The figure shows three views and two pictorial views of one solid part (mm, origin at its lowest corner). Answer the questions. A direction names the side the tool comes from. Round coordinates to 2 decimals unless told otherwise and drop trailing zeros. Order: outer loops, then holes, each group sorted by start corner. A loop starts at its lowest first (then second) coordinate and runs counter-clockwise, first axis right, second up. Notation, with made-up numbers: (60.25, 1) -> (97.25, 1) arc R14 cw to (97.25, 17) -> close; hole circle Ø9 at (9.5, 12.5). An arc over 180 degrees is marked (long way). Return JSON: item names as keys, results as strings. Group by question number.
(1) The part is cut by section B-B (z = 17.75). Determine the outline of the cut face in (x, y).
(2) The part is cut by section A-A (y = 67.5). Count the separate pieces of the cut face and the enclosed holes in it, plus the area to 3 significant figures.
(3) Consider line 1 (X direction, y = 57.15, z = 13.5); line 2 (Y direction, x = 19.05, z = 12.25); line 3 (Y direction, x = 37.5, z = 1.5). Determine where each line is inside the solid, lowest interval first. Write a range as [from, to].
(4) Each of these flat-tipped pins is pushed along its axis until it touches: pin 1 (10 mm diameter, centred on y = 40.5, z = 6, fed in from -X); pin 2 (15 mm diameter, centred on x = 19.05, y = 57.15, fed in from +Z); pin 3 (1.6 mm diameter, centred on y = 31.5, z = 1.5, fed in from +X); pin 4 (17 mm diameter, centred on x = 57, y = 32.5, fed in from -Z) (3 decimals). Where does it stop, or does it pass through?
(5) Which of the six approach directions +Z, -Z, +X, -X, +Y, -Y give full straight-line access (tool end or side, diameter ignored) to the marked faces 1 and 2?
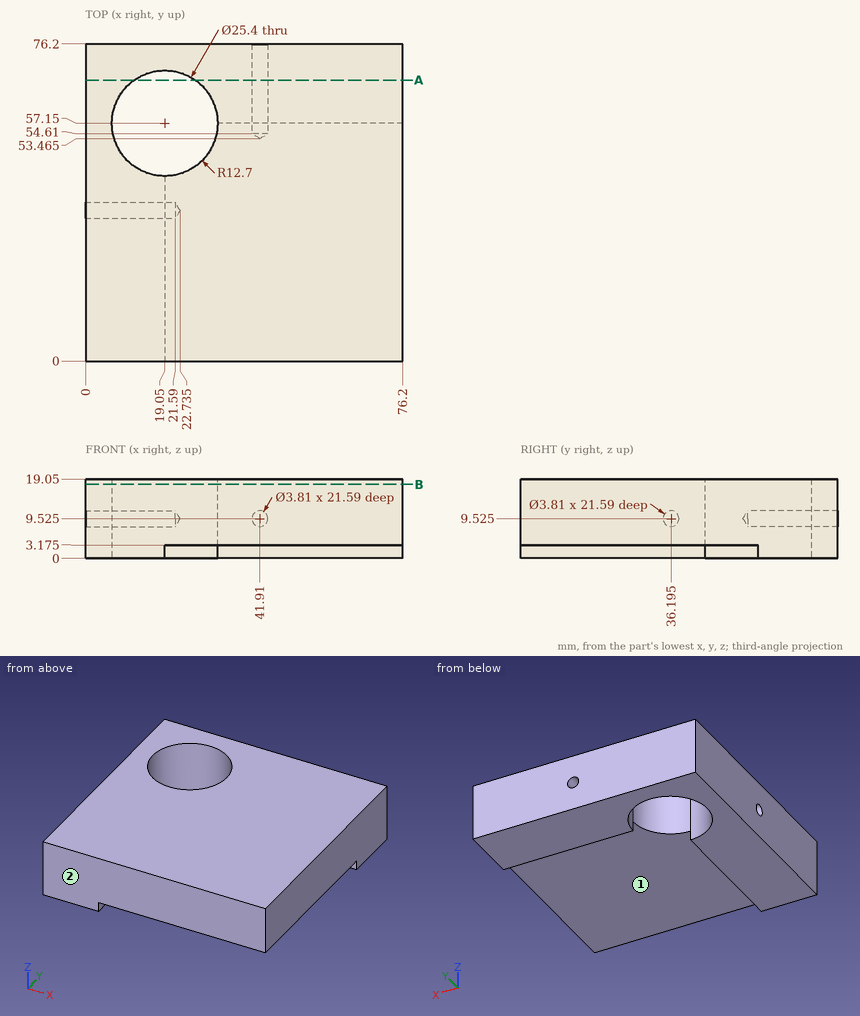
Answer below:
{
 "1": {"outline": "(0, 0) -> (76.2, 0) -> (76.2, 76.2) -> (0, 76.2) -> close; hole circle Ø25.4 at (19.05, 57.15)"},
 "2": {"separate pieces": "2", "enclosed holes": "1", "area": "1,160 mm²"},
 "3": {"line 1": "x = [0, 6.35], [31.75, 76.2]", "line 2": "y = [0, 44.45], [69.85, 76.2]", "line 3": "y = [57.15, 76.2]"},
 "4": {"pin 1": "stops at x = 0", "pin 2": "passes through", "pin 3": "stops at x = 19.05", "pin 4": "stops at z = 3.175"},
 "5": {"face 1": "-Z, +X, -Y", "face 2": "+Z, -Z, +X, -X, -Y"}
}
